from build123d import *

# Parameters (mm, degrees)
SKETCH1_W            = 127
SKETCH1_H            = 91.44
BOSS_EXTRUDE1_DEPTH  = 228.6
SKETCH3_W            = 120.65
SKETCH3_H            = 85.09
CUT_EXTRUDE1_DEPTH   = 226.06
SKETCH2_R            = 2.667
CUT_EXTRUDE2_DEPTH   = 266.475570251
SKETCH4_R            = 1.143
BOSS_EXTRUDE3_DEPTH  = 5.08
SKETCH5_R            = 20.32
CUT_EXTRUDE3_DEPTH   = 1.27
FILLET1_R            = 0.762
FILLET2_R            = 0.762
FILLET3_R            = 0.762
SKETCH6_W            = 60.96
SKETCH6_H            = 25.4
CUT_EXTRUDE4_DEPTH   = 256.582569828
FILLET4_R            = 2.54
SKETCH7_W            = 85.09
SKETCH7_H            = 111.152565629
CUT_EXTRUDE5_DEPTH   = 268.942913323
SKETCH10_R           = 2.667
CUT_EXTRUDE6_DEPTH   = 2.54
CUT_EXTRUDE7_DEPTH   = 7.62
SKETCH13_R           = 2.667
CUT_EXTRUDE8_DEPTH   = 2.54
CUT_EXTRUDE9_DEPTH   = 7.62
SKETCH20_W           = 11.43
SKETCH20_H           = 7.62
BOSS_EXTRUDE4_DEPTH  = 50.8
CUT_EXTRUDE10_START  = -12.7
SKETCH21_R           = 2.667
CUT_EXTRUDE10_DEPTH  = 12.7
CUT_EXTRUDE11_DEPTH  = 12.7
SKETCH24_R           = 3.81
BOSS_EXTRUDE5_DEPTH  = 3.81
SKETCH25_R           = 2.667
CUT_EXTRUDE12_DEPTH  = 3.81
CUT_EXTRUDE13_DEPTH  = 12.7
CUT_EXTRUDE14_START  = 64.77
SKETCH27_R           = 2.667
CUT_EXTRUDE14_DEPTH  = 64.77
CUT_EXTRUDE15_START  = 64.77
SKETCH29_R           = 2.667
CUT_EXTRUDE15_DEPTH  = 64.77
FILLET6_R            = 50.8
FILLET7_R            = 50.8
BOSS_EXTRUDE6_DEPTH  = 5.08
MIRROR5_COPY_1_DEPTH = 5.08
MIRROR6_COPY_1_DEPTH = 5.08
MIRROR6_COPY_2_DEPTH = 5.08
MIRROR6_COPY_3_DEPTH = 5.08


with BuildPart() as part:
    # Sketch1 → Boss-Extrude1 (new body)
    with BuildSketch(Plane(origin=(0, 0, 0), x_dir=(1, 0, 0), z_dir=(0, 1, 0))):
        Rectangle(SKETCH1_W, SKETCH1_H)
    extrude(amount=BOSS_EXTRUDE1_DEPTH)

    # Sketch3 → Cut-Extrude1 (cut)
    with BuildSketch(Plane.XZ):
        Rectangle(SKETCH3_W, SKETCH3_H)
    extrude(amount=-CUT_EXTRUDE1_DEPTH, mode=Mode.SUBTRACT)

    # Sketch2 → Cut-Extrude2 (cut, through all)
    with BuildSketch(Plane(origin=(63.5, 0, 0), x_dir=(0, 0, -1), z_dir=(1, 0, 0))):
        with Locations((0, 182.88)):
            Circle(SKETCH2_R)
    extrude(amount=-CUT_EXTRUDE2_DEPTH, mode=Mode.SUBTRACT)

    # Sketch4 → Boss-Extrude3 (add)
    with BuildSketch(Plane(origin=(63.5, 0, 0), x_dir=(0, 0, -1), z_dir=(1, 0, 0))):
        with Locations(Location((-40.64, 223.52, 0), (0, 0, 180))):
            Circle(SKETCH4_R)
        with Locations(Location((40.64, 223.52, 0), (0, 0, 180))):
            Circle(SKETCH4_R)
        with Locations(Location((40.64, 142.24, 0), (0, 0, 180))):
            Circle(SKETCH4_R)
        with Locations(Location((-40.64, 142.24, 0), (0, 0, 180))):
            Circle(SKETCH4_R)
    boss_extrude3 = extrude(amount=BOSS_EXTRUDE3_DEPTH)

    # Sketch5 → Cut-Extrude3 (cut)
    with BuildSketch(Plane.ZY.offset(-60.325)):
        with Locations((0, 182.88)):
            Circle(SKETCH5_R)
    cut_extrude3 = extrude(amount=-CUT_EXTRUDE3_DEPTH, mode=Mode.SUBTRACT)

    # Fillet1
    fillet1_edges = [part.edges().sort_by_distance(p)[0] for p in [
        (61.595, 182.88, 2.667),
    ]]
    fillet(fillet1_edges, radius=FILLET1_R)

    # Fillet2
    fillet2_edges = [part.edges().sort_by_distance(p)[0] for p in [
        (63.5, 182.88, 2.667),
    ]]
    fillet(fillet2_edges, radius=FILLET2_R)

    # Mirror2: Boss-Extrude3, Cut-Extrude3 across plane
    add(boss_extrude3.mirror(Plane(origin=(0, 0, 0), x_dir=(0, 0, 1), z_dir=(1, 0, 0))))
    add(cut_extrude3.mirror(Plane(origin=(0, 0, 0), x_dir=(0, 0, 1), z_dir=(1, 0, 0))), mode=Mode.SUBTRACT)

    # Fillet3
    fillet3_edges = [part.edges().sort_by_distance(p)[0] for p in [
        (-63.5, 182.88, 2.667),
        (-61.595, 182.88, 2.667),
    ]]
    fillet(fillet3_edges, radius=FILLET3_R)

    # Sketch6 → Cut-Extrude4 (cut, through all)
    with BuildSketch(Plane.XY.offset(45.72)):
        with Locations((0, 182.88)):
            Rectangle(SKETCH6_W, SKETCH6_H)
    extrude(amount=-CUT_EXTRUDE4_DEPTH, mode=Mode.SUBTRACT)

    # Fillet4
    fillet4_edges = [part.edges().sort_by_distance(p)[0] for p in [
        (-63.5, 228.6, 0),
        (0, 228.6, 45.72),
        (63.5, 228.6, 0),
        (63.5, 114.3, 45.72),
        (-63.5, 114.3, 45.72),
        (-63.5, 114.3, -45.72),
        (63.5, 114.3, -45.72),
        (0, 228.6, -45.72),
    ]]
    fillet(fillet4_edges, radius=FILLET4_R)

    # Sketch7 → Cut-Extrude5 (cut, through all)
    with BuildSketch(Plane(origin=(63.5, 0, 0), x_dir=(0, 0, -1), z_dir=(1, 0, 0))):
        with Locations((0, 75.896282814)):
            Rectangle(SKETCH7_W, SKETCH7_H)
    extrude(amount=-CUT_EXTRUDE5_DEPTH, mode=Mode.SUBTRACT)

    # Sketch10 → Cut-Extrude6 (cut)
    with BuildSketch(Plane.ZY.offset(-60.325)):
        with Locations((-30.48, 182.88)):
            Circle(SKETCH10_R)
    extrude(amount=-CUT_EXTRUDE6_DEPTH, mode=Mode.SUBTRACT)

    # Sketch12 → Cut-Extrude7 (cut)
    with BuildSketch(Plane(origin=(0, 0, -45.72), x_dir=(-1, 0, 0), z_dir=(0, 0, -1))):
        Polygon((-34.810362372, 182.807903476), (-34.810362372, 200.587903476), (-60.210362372, 200.587903476), (-60.210362372, 182.807903476), (-60.210362372, 165.027903476), (-34.810362372, 165.027903476), align=None)
    extrude(amount=-CUT_EXTRUDE7_DEPTH, mode=Mode.SUBTRACT)

    # Sketch13 → Cut-Extrude8 (cut)
    with BuildSketch(Plane(origin=(-60.325, 0, 0), x_dir=(0, 0, -1), z_dir=(1, 0, 0))):
        with Locations((-30.48, 182.88)):
            Circle(SKETCH13_R)
    extrude(amount=-CUT_EXTRUDE8_DEPTH, mode=Mode.SUBTRACT)

    # Sketch16 → Cut-Extrude9 (cut)
    with BuildSketch(Plane.XY.offset(45.72)):
        Polygon((-60.34639287, 182.934228321), (-60.34639287, 200.714228321), (-34.94639287, 200.714228321), (-34.94639287, 165.154228321), (-60.34639287, 165.154228321), align=None)
    extrude(amount=-CUT_EXTRUDE9_DEPTH, mode=Mode.SUBTRACT)

    # Sketch20 → Boss-Extrude4 (add)
    with BuildSketch(Plane.XZ.offset(-226.06)):
        with Locations((1.27, -30.48)):
            Rectangle(SKETCH20_W, SKETCH20_H)
    boss_extrude4 = extrude(amount=BOSS_EXTRUDE4_DEPTH)

    # Sketch21 → Cut-Extrude10 (cut)
    with BuildSketch(Plane(origin=(6.985, 0, 0), x_dir=(0, 0, -1), z_dir=(1, 0, 0)).offset(CUT_EXTRUDE10_START)):
        with Locations(Location((30.48, 182.88, 0), (0, 0, 180))):
            Circle(SKETCH21_R)
    cut_extrude10 = extrude(amount=CUT_EXTRUDE10_DEPTH, mode=Mode.SUBTRACT)

    # Sketch23 → Cut-Extrude11 (cut)
    with BuildSketch(Plane(origin=(6.985, 0, 0), x_dir=(0, 0, -1), z_dir=(1, 0, 0))):
        Polygon((27.813, 182.88), (26.67, 182.88), (26.67, 175.26), (34.29, 175.26), (34.29, 182.88), align=None)
    extrude(amount=-CUT_EXTRUDE11_DEPTH, mode=Mode.SUBTRACT)

    # Sketch24 → Boss-Extrude5 (add)
    with BuildSketch(Plane.ZY.offset(-30.48)):
        with Locations((-46.355, 182.88)):
            Circle(SKETCH24_R)
    boss_extrude5 = extrude(amount=-BOSS_EXTRUDE5_DEPTH)

    # Sketch25 → Cut-Extrude12 (cut)
    with BuildSketch(Plane.ZY.offset(-30.48)):
        with Locations((-46.355, 182.88)):
            Circle(SKETCH25_R)
    cut_extrude12 = extrude(amount=-CUT_EXTRUDE12_DEPTH, mode=Mode.SUBTRACT)

    # Mirror3: Boss-Extrude4, Cut-Extrude10, Boss-Extrude5, Cut-Extrude12 across plane
    add(boss_extrude4.mirror(Plane.XY))
    add(cut_extrude10.mirror(Plane.XY), mode=Mode.SUBTRACT)
    add(boss_extrude5.mirror(Plane.XY))
    add(cut_extrude12.mirror(Plane.XY), mode=Mode.SUBTRACT)

    # Sketch26 → Cut-Extrude13 (cut)
    with BuildSketch(Plane(origin=(6.985, 0, 0), x_dir=(0, 0, -1), z_dir=(1, 0, 0))):
        Polygon((-27.813, 182.88), (-26.67, 182.88), (-26.67, 175.26), (-34.29, 175.26), (-34.29, 182.88), align=None)
    extrude(amount=-CUT_EXTRUDE13_DEPTH, mode=Mode.SUBTRACT)

    # Sketch27 → Cut-Extrude14 (cut)
    with BuildSketch(Plane.ZY.offset(-30.48).offset(CUT_EXTRUDE14_START)):
        with Locations((-46.355, 182.88)):
            Circle(SKETCH27_R)
    extrude(amount=-CUT_EXTRUDE14_DEPTH, mode=Mode.SUBTRACT)

    # Sketch29 → Cut-Extrude15 (cut)
    with BuildSketch(Plane.ZY.offset(-30.48).offset(CUT_EXTRUDE15_START)):
        with Locations(Location((46.355, 182.88, 0), (0, 0, 256.225853002))):
            Circle(SKETCH29_R)
    extrude(amount=-CUT_EXTRUDE15_DEPTH, mode=Mode.SUBTRACT)

    # Fillet6
    # the kernel refuses this fillet: 50.8 mm, written as the material it takes off along each edge
    with BuildSketch(Plane(origin=(33.773797915, 182.88, 34.29), x_dir=(0, 0, -1), z_dir=(-1, 0, 0))) as fillet6_piece_1:
        with BuildLine():
            CenterArc((50.8, -10.715519166), FILLET6_R, 167.822824326, 12.177175674)
            Line((0, -10.715519166), (-1.016, -10.715519166))
            Line((-1.016, -10.715519166), (-1.016, 0))
            Line((-1.016, 0), (0, 1.016))
            ThreePointArc((0, 1.016), (0.5715, 1.016), (0.14986, 0.214310383))
            Line((0.14986, 0.214310383), (1.143, 0))
        make_face()
    extrude(amount=65.007595831, mode=Mode.SUBTRACT)

    # Fillet7
    # the kernel refuses this fillet: 50.8 mm, written as the material it takes off along each edge
    with BuildSketch(Plane(origin=(33.773797915, 182.88, -34.29), x_dir=(0, 1, 0), z_dir=(-1, 0, 0))) as fillet7_piece_1:
        with BuildLine():
            CenterArc((10.715519166, -50.8), FILLET7_R, 90, 12.177175674)
            Line((0, -1.143), (0, 0))
            Line((0, 0), (10.715519166, 0))
        make_face()
    extrude(amount=65.007595831, mode=Mode.SUBTRACT)

    # Sketch33 → Boss-Extrude6 (add)
    with BuildSketch(Plane(origin=(0, 228.6, 0), x_dir=(1, 0, 0), z_dir=(0, 1, 0))):
        Polygon((63.5, 43.18), (63.5, 50.8), (58.42, 50.8), (58.42, 48.26), (60.96, 48.26), (60.96, 43.18), align=None)
    boss_extrude6 = extrude(amount=-BOSS_EXTRUDE6_DEPTH)

    # Mirror4: Boss-Extrude6 across plane
    add(boss_extrude6.mirror(Plane(origin=(0, 0, 0), x_dir=(0, 0, 1), z_dir=(1, 0, 0))))

    # Mirror5: Boss-Extrude6 across plane
    add(boss_extrude6.mirror(Plane.ZX.offset(182.88)))

    # Mirror5 copy 1 sketch → Mirror5 copy 1 (add)
    with BuildSketch(Plane(origin=(0, 137.16, 0), x_dir=(-1, 0, 0), z_dir=(0, -1, 0))):
        Polygon((63.5, 43.18), (63.5, 50.8), (58.42, 50.8), (58.42, 48.26), (60.96, 48.26), (60.96, 43.18), align=None)
    extrude(amount=-MIRROR5_COPY_1_DEPTH)

    # Mirror6: Boss-Extrude6 across plane
    add(boss_extrude6.mirror(Plane.XY))

    # Mirror6 copy 1 sketch → Mirror6 copy 1 (add)
    with BuildSketch(Plane(origin=(0, 228.6, 0), x_dir=(-1, 0, 0), z_dir=(0, 1, 0))):
        Polygon((63.5, 43.18), (63.5, 50.8), (58.42, 50.8), (58.42, 48.26), (60.96, 48.26), (60.96, 43.18), align=None)
    extrude(amount=-MIRROR6_COPY_1_DEPTH)

    # Mirror6 copy 2 sketch → Mirror6 copy 2 (add)
    with BuildSketch(Plane.XZ.offset(-137.16)):
        Polygon((63.5, 43.18), (63.5, 50.8), (58.42, 50.8), (58.42, 48.26), (60.96, 48.26), (60.96, 43.18), align=None)
    extrude(amount=-MIRROR6_COPY_2_DEPTH)

    # Mirror6 copy 3 sketch → Mirror6 copy 3 (add)
    with BuildSketch(Plane(origin=(0, 137.16, 0), x_dir=(-1, 0, 0), z_dir=(0, -1, 0))):
        Polygon((63.5, -43.18), (63.5, -50.8), (58.42, -50.8), (58.42, -48.26), (60.96, -48.26), (60.96, -43.18), align=None)
    extrude(amount=-MIRROR6_COPY_3_DEPTH)


solid = part.part
Can you work these out from the model? Positions are in its coordinate system, mm. A direction names the side the tool comes from. Coordinates: 2 decimals unless noted, no trailing zeros. Write each loop counter-clockwise with the first axis right and the second up, starting at its lowest first coordinate (ties: lowest second). Pieces come first, ordered by that corner, then holes. Notation, with made-up numbers: (85.25, 10) - (92.25, 10) arc R12 ccw to (92.25, 19) - close; hole circle Ø3 at (46, -21.75). An arc over 180 degrees is marked (long way). Return JSON: item names as keys, results as strings. Group by question number.
Item 1: We'd pull the mould along Z, two halves only. Please class faces 1 (the face through (1.35, 188.132, 33.995)), 2 (the face through (60.96, 226, 47)), 3 (the face through (61, 142.24, -49)): pulls with the +Z half, pulls with the -Z half, needs draft (parallel to the pull), parting line crosses it, or undercut.
Item 2: I'm going to push flat-ended pins straight in: pin 1 Ø1.5 at (x, y) = (52, 133) entering from +Z; pin 2 Ø0.6 at (y, z) = (182, -44.5) entering from +X; pin 3 Ø1.3 at (y, z) = (183.5, -47) entering from +X; pin 4 Ø22.5 at (y, z) = (9.5, 5) entering from -X. Where does each tip first touch, or does it pass through?
Item 3: Which directions (+Z, -Z, +X, -X, +Y, -Y) give clear straight access to the entire face, cutting with the end or side of a thin tool? Please do faces 4 (the face through (-61.577, 183.681, 27.936)), 5 (the face through (30.48, 183, -43)), 6 (the face through (-60.325, 157, -1)).
Item 4: If we section it at B-B (y = 72): Write out the boundary of the cut face in (x, z) (3 decimals), then the cut area to 3 significant figures.
Item 5: If we section it at C-C (x = 46.5): Write out the boundary of the cut face in (y, z) (3 decimals), then the cut area to 3 significant figures.
Item 6: Please list where these lines run through material, in increasing order: probe 1 along X at (y, z) = (156.5, 20) (3 decimals); probe 2 along Z at (x, y) = (62.55, 182.88); probe 3 along Y at (x, z) = (-61.65, 30.48).
Item 7: If we section it at D-D (x = 4.5): Count the separate pieces of the cut face and the enclosed holes in it, then the cut area to 3 significant figures.
Item 8: If we section it at A-A (z = 30.48): Write out the boundary of the cut face in (x, y) (3 decimals), then the cut area to 3 significant figures.
Return value:
{
 "1": {"face 1": "pulls with the +Z half", "face 2": "undercut", "face 3": "needs draft"},
 "2": {"pin 1": "stops at z = 45.72", "pin 2": "stops at x = 63.29", "pin 3": "passes through", "pin 4": "stops at x = -63.5"},
 "3": {"face 4": "none", "face 5": "+Z, -Z", "face 6": "-Y"},
 "4": {"outline": "(-63.5, -43.18) arc R2.54 ccw to (-60.96, -45.72) - (60.96, -45.72) arc R2.54 ccw to (63.5, -43.18) - (63.5, -42.545) - (-63.5, -42.545) - close; (-63.5, 42.545) - (63.5, 42.545) - (63.5, 43.18) arc R2.54 ccw to (60.96, 45.72) - (-60.96, 45.72) arc R2.54 ccw to (-63.5, 43.18) - close", "area": "801 mm^2"},
 "5": {"outline": "(0, -45.72) - (165.028, -45.72) - (165.028, -42.545) - (0, -42.545) - close; (0, 42.545) - (226.06, 42.545) - (226.06, -42.545) - (200.588, -42.545) - (200.588, -45.72) - (226.06, -45.72) arc R2.54 ccw to (228.6, -43.18) - (228.6, 43.18) arc R2.54 ccw to (226.06, 45.72) - (0, 45.72) - close", "area": "1,550 mm^2"},
 "6": {"probe 1": "x = -63.5 to -60.325, 60.325 to 63.5", "probe 2": "z = -45.16 to -33.15, -27.81 to -2.67, 2.67 to 45.16", "probe 3": "y = 0 to 20.32, 131.47 to 180.21, 185.55 to 228.5"},
 "7": {"separate pieces": "3", "enclosed holes": "0", "area": "2,130 mm^2"},
 "8": {"outline": "(-63.5, 0) - (-60.325, 0) - (-60.325, 20.32) - (-63.5, 20.32) - close; (-63.5, 131.473) - (-60.325, 131.473) - (-60.325, 180.213) - (-62.865, 180.213) - (-62.865, 185.547) - (-60.325, 185.547) - (-60.325, 226.06) - (-4.445, 226.06) - (-4.445, 185.547) - (6.985, 185.547) - (6.985, 226.06) - (60.325, 226.06) - (60.325, 131.473) - (63.5, 131.473) - (63.5, 226.06) arc R2.54 ccw to (60.96, 228.6) - (-60.96, 228.6) arc R2.54 ccw to (-63.5, 226.06) - close; (60.325, 0) - (63.5, 0) - (63.5, 20.32) - (60.325, 20.32) - close", "area": "1,500 mm^2"}
}
